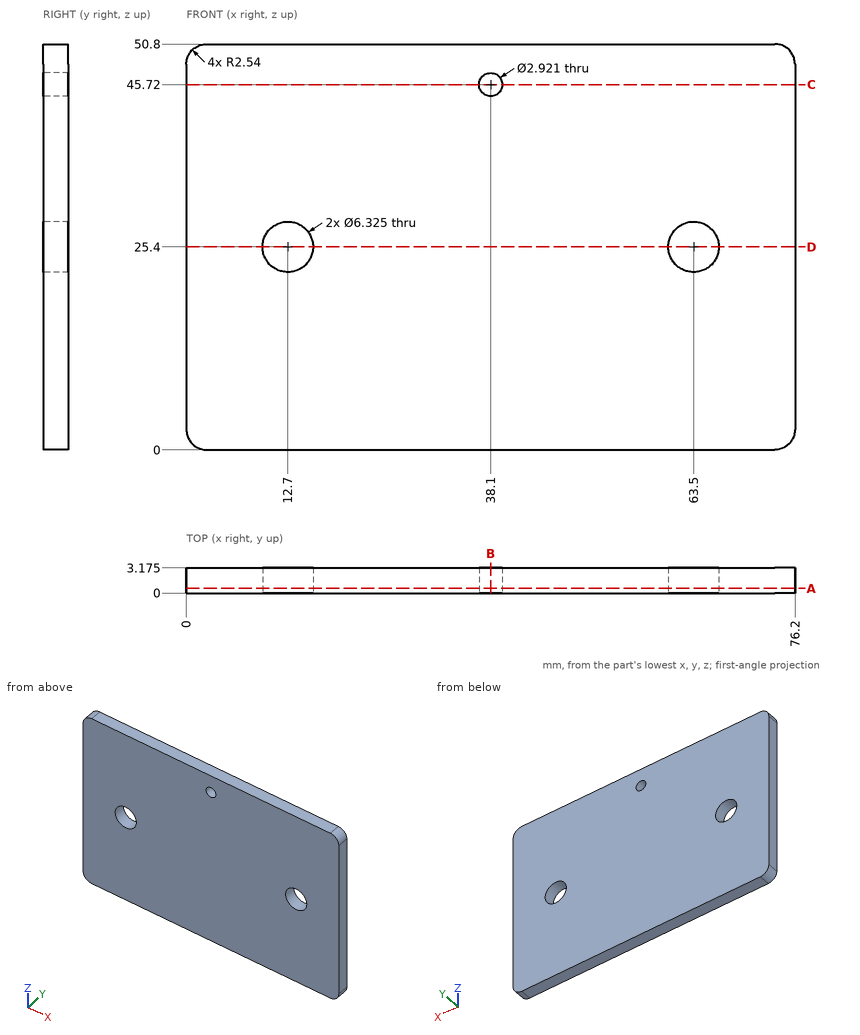
Source: three-view drawing plus pictorial views. Frame: mm from the lowest corner of the part. Round coordinates to 2 decimals unless told otherwise and drop trailing zeros. Loops run counter-clockwise (first coordinate to the right, second up) from the corner with the lowest first, then second, coordinate; pieces in that order, holes last. Notation, with made-up numbers: (81, 38.25) - (117, 38.25) arc R21 cw to (117, 43.25) - close; hole circle Ø3 at (11.5, -11.75). An arc over 180 degrees is marked (long way). Write item = value, one per line. Start each with the question number.
Item 1: Section query A-A on y = 0.6. Output: boundary loops of the cut face in (x, z) (1 decimal).
Item 2: Material intervals for line 1 (X direction, y = 1.95, z = 25.4); line 2 (Z direction, x = 38.1, y = 2.4); line 3 (X direction, y = 1.85, z = 45.72), sorted ascending.
Item 3: Section query B-B on x = 38.1. Output: boundary loops of the cut face in (y, z) (1 decimal), plus the area to 3 significant figures.
Item 4: Section query D-D on z = 25.4. Output: boundary loops of the cut face in (x, y) (1 decimal), plus the area to 3 significant figures.
Item 5: Section query C-C on z = 45.72. Output: boundary loops of the cut face in (x, y) (1 decimal).
Results list:
q1.outline = (0, 2.5) arc R2.5 ccw to (2.5, 0) - (73.7, 0) arc R2.5 ccw to (76.2, 2.5) - (76.2, 48.3) arc R2.5 ccw to (73.7, 50.8) - (2.5, 50.8) arc R2.5 ccw to (0, 48.3) - close; hole circle Ø6.3 at (12.7, 25.4); hole circle Ø2.9 at (38.1, 45.7); hole circle Ø6.3 at (63.5, 25.4)
q2.line_1 = 0 to 9.54, 15.86 to 60.34, 66.66 to 76.2
q2.line_2 = 0 to 44.26, 47.18 to 50.8
q2.line_3 = 0 to 36.64, 39.56 to 76.2
q3.outline = (0, 0) - (3.2, 0) - (3.2, 44.3) - (0, 44.3) - close; (0, 47.2) - (3.2, 47.2) - (3.2, 50.8) - (0, 50.8) - close
q3.area = 152 mm²
q4.outline = (0, 0) - (9.5, 0) - (9.5, 3.2) - (0, 3.2) - close; (15.9, 0) - (60.3, 0) - (60.3, 3.2) - (15.9, 3.2) - close; (66.7, 0) - (76.2, 0) - (76.2, 3.2) - (66.7, 3.2) - close
q4.area = 202 mm²
q5.outline = (0, 0) - (36.6, 0) - (36.6, 3.2) - (0, 3.2) - close; (39.6, 0) - (76.2, 0) - (76.2, 3.2) - (39.6, 3.2) - close
